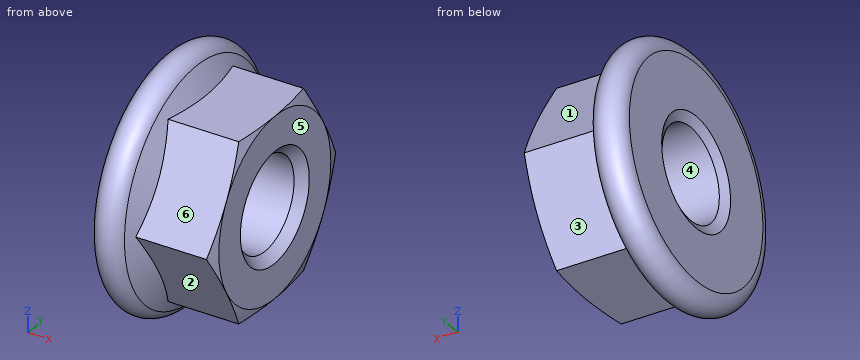
Autodesk Inventor part; units mm, degrees
ref_plane "Work Plane1" through (26.5484, 0, 0) normal (0, 0, -1) x (-1, 0, 0)
ref_plane "YZ Plane" through (0, 0, 0) normal (1, 0, 0) x (0, 1, 0)
ref_plane "XZ Plane" through (0, 0, 0) normal (0, 1, 0) x (-1, 0, 0)
sketch "Sketch1" plane through (0, 0, 0) normal (0, 0, 1) x (1, 0, 0)
  line L0 (-1.8442, 0) -> (9.6407, 0)
  line L1 (3.1069, 6.5) -> (2.2876, 8.2571)
  line L2 (3.1069, 6.5) -> (8, 6.5) construction
  line L3 (8, 6.5) -> (8, 0) construction
  arc A0 (2.2876, 8.2571) -> (0, 7.75) centre (1.2, 7.75) ccw
  line L4 (3.1069, 6.5) -> (3.1069, 0)
  line L5 (0, -1.835) -> (0, 11.0102)
  point P0 (0, 0)
  dimension "d2" = 13
  dimension "d4" = 17.9
  dimension "d5" = 1.2
  dimension "d15" = 8
  dimension "d16" = 25
revolve "Ring" add sketch "Sketch1" angle 360 about axis through (-10, 0, 0) along (1, 0, 0)
sketch "Sketch2" plane through (0, 0, 0) normal (-1, 0, 0) x (0, 0, 1)
  circle A0 centre (0, 0) radius 4.9
  line L0 (-6.5, -3.7528) -> (-6.5, 3.7528)
  line L1 (-6.5, 3.7528) -> (0, 7.5056)
  line L2 (0, 7.5056) -> (6.5, 3.7528)
  line L3 (6.5, 3.7528) -> (6.5, -3.7528)
  line L4 (6.5, -3.7528) -> (0, -7.5056)
  line L5 (0, -7.5056) -> (-6.5, -3.7528)
  circle A1 centre (0, 0) radius 7.75
  dimension "d6" = 15.0111
extrude "Body" add sketch "Sketch2" against normal blind 8 contours A0 | L0 L1 L2 L3 L4 L5
sketch "Sketch3" plane through (0, 0, 0) normal (0, 0, 1) x (1, 0, 0)
  line L0 (2.638, 7.5056) -> (8, 7.5056)
  line L1 (8, 3.7528) -> (8, 7.5056)
  line L2 (0, -7.75) -> (0, 7.75)
  line L3 (-1.6, 0) -> (9.6, 0)
  line L4 (7.7306, 7.5056) -> (8, 6.5)
  dimension "d10" = 15
  dimension "d11" = 13
revolve "Chamfer1" cut sketch "Sketch3" angle 360 about axis through (-10, 0, 0) along (1, 0, 0)
sketch "Sketch4" plane through (0, 0, 0) normal (-1, 0, 0) x (0, 0, 1)
  circle A0 centre (0, 0) radius 7.75
hole "Thread" at (0, 0, 0) direction (1, 0, 0) diameter 6.647 end through all
chamfer "Chamfer2" distance 0.6766 angle 30 1 edges at (0, 0, -3.3235) measured on face at (0, 6.1914, -0.7518)
ref_plane "Work Plane1" through (26.5484, 0, 0) normal (0, 0, -1) x (-1, 0, 0)
chamfer "Chamfer3" distance 0.6766 angle 45 1 edges at (8, 0, -3.3235)
equation "\"d2\" = SW"
equation "\"d4\" = LADI"
equation "\"d5\" = PHH"
equation "\"d15\" = KOH"
equation "\"d16\" = KEWI"
equation "\"d6\" = 1.1547 * SW"
equation "\"d7\" = KOH"
equation "\"d10\" = ANG1"
equation "\"d11\" = SW0"
equation "\"d12\" = -0.5 * GD1 + 0.5 * NND"
equation "\"d46\" = -0.5 * GD1 + 0.5 * NND"
equation "\"d51\" = -0.5 * GD1 + 0.5 * NND"
equation "\"ANG1\" = 15deg"
equation "\"KEWI\" = 25deg"
equation "\"NND\" = 8"
equation "\"LADI\" = 17.9"
equation "\"SW\" = 13"
equation "\"PHH\" = RR"
equation "\"KOH\" = NND"
equation "\"SW0\" = SW"
equation "\"d1\" = LADI"
equation "\"d3\" = PHH"
equation "\"GUL\" = 0.541266 * PTC"
equation "\"RR\" = 1.2"
equation "\"THREADDIA\" = 8"
equation "\"TOA\" = 30deg"
equation "\"PTC\" = 1.25"
equation "\"GAL\" = 0.541266 * PTC"
equation "\"E0\" = 1.155 * SW"
properties part number "DIN 6923 - M8" material "Steel, Mild"
Build history of the part. All positions in model axes, mm. Face numbers are marked on the shaded views. A direction names the side the tool comes from. Coordinates: 2 decimals unless noted, no trailing zeros. Order: outer loops, then holes, each group sorted by start corner. A loop starts at its lowest first (then second) coordinate and runs counter-clockwise, first axis right, second up. Notation, with made-up numbers: M -39,10.5 L 9,10.5 A18 ccw 9,30.5 Z; hole C 1,51 d9. An arc over 180 degrees is marked long. One line per question, with ' | ' between items. Start each with the question number.
1. Mould opens along Y. For the marked faces 4, 5 and 6 say: +Y half, -Y half, draft (parallel to the pull), parting line (faces both ways), or undercut.
2. Cut at A-A (x = 5). Write the cut outline in (y, z), plus the area to 3 significant figures.
3. Flat gauge pins, fed straight in: P1, Ø2.5, axis at x = 4, y = -1, coming from the -Z side; P2, Ø3, axis at x = 6.5, z = -2, coming from the -Y side; P3, Ø4, axis at y = -6, z = -7, coming from the +X side; P4, Ø6, axis at y = 0, z = 0, coming from the +X side. Where does each tip first touch, or does it go through?
4. Tool access for the marked faces 1, 2 and 3: list every direction of +Z, -Z, +X, -X, +Y, -Y with a clear straight run to the whole face (end or side of a thin tool).
5. Cut at B-B (x = 1). Write the cut outline in (y, z), plus the area to 3 significant figures.
6. Wall check: line 1 along Z through (x, y) = (4.5, 0); line 2 along Y through (x, z) = (6, 0.5); line 3 along Y through (x, z) = (6, -2). Give the ranges that are in metal, low to high. Write a range as [from, to].
The answers:
1) face 4: undercut | face 5: draft | face 6: -Y half
2) outline: M -7.51,0 L -3.75,-6.5 L 3.75,-6.5 L 7.51,0 L 3.75,6.5 L -3.75,6.5 Z; hole C 0,0 d6.65 | area: 112 mm2
3) P1: stops at z = -7.2 | P2: stops at y = -7.22 | P3: stops at x = 2.77 | P4: passes through
4) face 1: +Z, +X, +Y | face 2: -Z, +X, -Y | face 3: -Z, +X, +Y
5) outline: C 0,0 d17.87; hole C 0,0 d6.65 | area: 216 mm2
6) line 1: z = [-6.5, -3.32], [3.32, 6.5] | line 2: y = [-7.22, -3.29], [3.29, 7.22] | line 3: y = [-6.35, -2.65], [2.65, 6.35]
